The model under review builds one solid part; all positions refer to its coordinate system, in mm. A direction names the side the tool comes from. Coordinates: 2 decimals unless noted, no trailing zeros. Write each loop counter-clockwise with the first axis right and the second up, starting at its lowest first coordinate (ties: lowest second). Pieces come first, ordered by that corner, then holes.
1) Mouldability with a two-part tool opening along Y and no side actions: class faces 1 (the flat face through (-57.486, 8, 27)), 2 (the cylindrical face through (-55.34, 41.02, 26.82)), 3 (the cylindrical face through (-51.366, 21.628, 25.64)), 4 (the flat face through (-44.7, 10.2, 24.9)) as released by +Y, released by -Y, zero draft, split by the parting line, or undercut.
2) Add section A-A, the plane x = -46. State the section outline as (y, z) points.
3) For P1, Ø2, axis at x = -52, y = -8.5, coming from the +Z side; P2, Ø1.9, axis at x = -51, z = 27, coming from the -Y side; P3, Ø2, axis at x = -28.5, z = 25.5, coming from the -Y side; P4, Ø5, axis at x = -51.24, y = -8.77, coming from the +Z side, all flat-tipped, find the tip position at first contact; note any pin that passes through.
4) Add section B-B, the plane y = 12. State the section outline as (x, z) points.
5) For line 1 (Y direction, x = -50, z = 26.7); line 2 (Y direction, x = -49, z = 25.8); line 3 (X direction, y = 5, z = 28.15), list the stretches that pass through material, from the lowest coordinate up.
6) Machinability: for faces 5 (the flat face through (-51, 17.587, 27)), 6 (the flat face through (-51, -10, 26.4)), 7 (the flat face through (-44.7, 10.2, 28.8)), which of the approach directions +Z, -Z, +X, -X, +Y, -Y give a long, thin tool a straight path to every point of the face, cutting with its end or side? Answer none if there is none.
7) Add section C-C, the plane z = 28.2. State the section outline as (x, y) points, then the cut area to 3 significant figures.
8) Add section D-D, the plane x = -28.5. State the section outline as (y, z) points, then the cut area to 3 significant figures.
from build123d import *

# Parameters (mm, degrees)
CROQUIS1_R              = 31.5
SALIENTE_EXTRUIR1_DEPTH = 2.4
CROQUIS2_W              = 16.1
CROQUIS2_H              = 36.6
CROQUIS2_W_2            = 12.5
CROQUIS2_H_2            = 33
SALIENTE_EXTRUIR2_DEPTH = 22.5
CROQUIS5_W              = 16.1
CROQUIS5_H              = 36.6
CORTAR_EXTRUIR2_DEPTH   = 9
CROQUIS6_R              = 1.5
CORTAR_EXTRUIR3_DEPTH   = 2.4
CROQUIS7_W              = 12.5
CROQUIS7_H              = 9
SALIENTE_EXTRUIR3_DEPTH = 33
CROQUIS8_R              = 1
CORTAR_EXTRUIR5_DEPTH   = 9
SALIENTE_EXTRUIR4_DEPTH = 12.5
CROQUIS10_W             = 4
CROQUIS10_H             = 2
CORTAR_EXTRUIR6_DEPTH   = 9
CROQUIS11_R             = 31.5
CROQUIS11_W             = 12.5
CROQUIS11_H             = 18
SALIENTE_EXTRUIR5_DEPTH = 3.9
CORTAR_EXTRUIR7_START   = 7
CROQUIS12_R             = 1
CORTAR_EXTRUIR7_DEPTH   = 3.9
CROQUIS13_R             = 2
CORTAR_EXTRUIR8_DEPTH   = 2.4
CROQUIS14_R             = 31.5
CORTAR_EXTRUIR9_DEPTH   = 24.9


with BuildPart() as part:
    # Croquis1 → Saliente-Extruir1 (new body)
    with BuildSketch(Plane.XY):
        with Locations((-51.235671923, 9.786589019)):
            Circle(CROQUIS1_R)
    extrude(amount=SALIENTE_EXTRUIR1_DEPTH)

    # Croquis2 → Saliente-Extruir2 (add)
    with BuildSketch(Plane.XY.offset(2.4)):
        with Locations((-51.235671923, 6.086589019)):
            Rectangle(CROQUIS2_W, CROQUIS2_H)
        with Locations((-51.235671923, 6.086589019)):
            Rectangle(CROQUIS2_W_2, CROQUIS2_H_2, mode=Mode.SUBTRACT)
    extrude(amount=SALIENTE_EXTRUIR2_DEPTH)

    # Croquis5 → Cortar-Extruir2 (cut)
    with BuildSketch(Plane.XY.offset(2.4)):
        with Locations((-51.235671923, 6.086589019)):
            Rectangle(CROQUIS5_W, CROQUIS5_H)
    extrude(amount=-CORTAR_EXTRUIR2_DEPTH, mode=Mode.SUBTRACT)


with BuildPart() as cortar_extruir2_piece_1:
    # of the separate pieces the step leaves, piece 1, a body of its own (cortar_extruir2_pieces)
    add(part.part.solids().sort_by_distance((-19.735671923, 9.786589019, 0))[0])

    # Croquis6 → Cortar-Extruir3 (cut)
    with BuildSketch(Plane(origin=(0, 0, 0), x_dir=(-1, 0, 0), z_dir=(0, 0, -1))):
        with Locations((34.618662565, 26.403598377)):
            Circle(CROQUIS6_R)
        with Locations((67.85268128, 26.403598377)):
            Circle(CROQUIS6_R)
        with Locations((67.85268128, -6.830420339)):
            Circle(CROQUIS6_R)
        with Locations((34.618662565, -6.830420339)):
            Circle(CROQUIS6_R)
        Polygon((51.235671923, 24.386589019), (53.235671923, 24.386589019), (53.235671923, 44.386589019), (49.235671923, 44.386589019), (49.235671923, 24.386589019), align=None)
    extrude(amount=-CORTAR_EXTRUIR3_DEPTH, mode=Mode.SUBTRACT)


with BuildPart() as cortar_extruir2_piece_2:
    # of the separate pieces the step leaves, piece 2, a body of its own (cortar_extruir2_pieces)
    add(part.part.solids().sort_by_distance((-59.285671923, -12.213410981, 24.9))[0])

    # Croquis7 → Saliente-Extruir3 (add)
    with BuildSketch(Plane.XZ.offset(-22.586589019)):
        with Locations((-51.235671923, 13.4)):
            Rectangle(CROQUIS7_W, CROQUIS7_H)
    extrude(amount=SALIENTE_EXTRUIR3_DEPTH)

    # Croquis8 → Cortar-Extruir5 (cut)
    with BuildSketch(Plane.XY.offset(17.9)):
        with Locations((-51.235671923, -8.413410981)):
            Circle(CROQUIS8_R)
        with Locations((-51.235671923, 20.636589019)):
            Circle(CROQUIS8_R)
        Polygon((-44.985671923, -5.413410981), (-57.485671923, -5.413410981), (-57.485671923, 17.586589019), (-53.235671923, 17.586589019), (-53.235671923, 19.586589019), (-49.235671923, 19.586589019), (-49.235671923, 17.586589019), (-44.985671923, 17.586589019), align=None)
    extrude(amount=-CORTAR_EXTRUIR5_DEPTH, mode=Mode.SUBTRACT)

    # Croquis9 → Saliente-Extruir4 (add)
    with BuildSketch(Plane.ZY.offset(44.985671923)):
        Polygon((8.9, -5.413410981), (3.9, -10.413410981), (8.9, -10.413410981), align=None)
        Polygon((8.9, 17.586589019), (3.9, 22.586589019), (8.9, 22.586589019), align=None)
    extrude(amount=SALIENTE_EXTRUIR4_DEPTH)

    # Croquis10 → Cortar-Extruir6 (cut)
    with BuildSketch(Plane.XY.offset(8.9)):
        with Locations((-51.235671923, 18.586589019)):
            Rectangle(CROQUIS10_W, CROQUIS10_H)
    extrude(amount=-CORTAR_EXTRUIR6_DEPTH, mode=Mode.SUBTRACT)

    # Croquis11 → Saliente-Extruir5 (add)
    with BuildSketch(Plane.XY.offset(24.9)):
        with Locations((-51.235671923, 9.786589019)):
            Circle(CROQUIS11_R)
        with Locations((-51.235671923, 8.586589019)):
            Rectangle(CROQUIS11_W, CROQUIS11_H, mode=Mode.SUBTRACT)
    extrude(amount=SALIENTE_EXTRUIR5_DEPTH)

    # Croquis12 → Cortar-Extruir7 (cut)
    with BuildSketch(Plane.XY.offset(17.9).offset(CORTAR_EXTRUIR7_START)):
        with Locations((-51.235671923, 20.636589019)):
            Circle(CROQUIS12_R)
        with Locations((-51.235671923, -8.413410981)):
            Circle(CROQUIS12_R)
    extrude(amount=CORTAR_EXTRUIR7_DEPTH, mode=Mode.SUBTRACT)

    # Croquis13 → Cortar-Extruir8 (cut)
    with BuildSketch(Plane.XY.offset(28.8)):
        with Locations((-51.235671923, 20.636589019)):
            Circle(CROQUIS13_R)
        with Locations((-51.235671923, -8.771160787)):
            Circle(CROQUIS13_R)
    extrude(amount=-CORTAR_EXTRUIR8_DEPTH, mode=Mode.SUBTRACT)


with BuildPart() as cortar_extruir9_tool:
    # Croquis14 → Cortar-Extruir9 (new body)
    with BuildSketch(Plane(origin=(0, 0, 0), x_dir=(-1, 0, 0), z_dir=(0, 0, -1))):
        with Locations(Location((51.235671923, 9.786589019, 0), (0, 0, 180))):
            Circle(CROQUIS14_R)
    extrude(amount=-CORTAR_EXTRUIR9_DEPTH)


with BuildPart() as cortar_extruir2_piece_1_1:
    add(cortar_extruir2_piece_1.part)

    # Cortar-Extruir9: cut by cortar_extruir9_tool
    add(cortar_extruir9_tool.part, mode=Mode.SUBTRACT)


with BuildPart() as cortar_extruir2_piece_2_1:
    add(cortar_extruir2_piece_2.part)

    # Cortar-Extruir9: cut by cortar_extruir9_tool
    add(cortar_extruir9_tool.part, mode=Mode.SUBTRACT)


solid = cortar_extruir2_piece_2_1.part
Geometry results:
1. face 1: undercut
1. face 2: split by the parting line
1. face 3: undercut
1. face 4: zero draft
2. outline: (-21.28, 24.9) - (-0.41, 24.9) - (-0.41, 28.8) - (-21.28, 28.8) - close; (17.59, 24.9) - (40.85, 24.9) - (40.85, 28.8) - (17.59, 28.8) - close
3. P1: stops at z = 26.4
3. P2: stops at y = -21.71
3. P3: stops at y = -13.01
3. P4: stops at z = 28.8
4. outline: (-82.66, 24.9) - (-57.49, 24.9) - (-57.49, 28.8) - (-82.66, 28.8) - close; (-44.99, 24.9) - (-19.81, 24.9) - (-19.81, 28.8) - (-44.99, 28.8) - close
5. line 1: y = -21.69 to -10.34, -7.2 to -0.41, 17.59 to 19.06, 22.21 to 41.26
5. line 2: y = -21.63 to -0.41, 17.59 to 41.21
5. line 3: x = -82.37 to -57.49, -44.99 to -20.1
6. face 5: +Z, -Z
6. face 6: +Z
6. face 7: +Z, +X, -X, +Y, -Y
7. outline: circle Ø63 at (-51.24, 9.79); hole (-57.49, -0.41) - (-44.99, -0.41) - (-44.99, 17.59) - (-57.49, 17.59) - close; hole circle Ø4 at (-51.24, -8.77); hole circle Ø4 at (-51.24, 20.64)
7. area: 2,870 mm2
8. outline: (-12.02, 24.9) - (31.59, 24.9) - (31.59, 28.8) - (-12.02, 28.8) - close
8. area: 170 mm2
